Here's how the part is built. I have some questions about the finished solid (model axes, mm). Face numbers are marked on the shaded views. A direction names the side the tool comes from. Round coordinates to 2 decimals unless told otherwise and drop trailing zeros. Write each loop counter-clockwise with the first axis right and the second up, starting at its lowest first coordinate (ties: lowest second). Pieces come first, ordered by that corner, then holes. Notation, with made-up numbers: (57.5, -28) -> (93.5, -28) arc R13 ccw to (93.5, -3) -> close; hole circle Ø1 at (-1.5, 34.25). An arc over 180 degrees is marked (long way). Answer in a Markdown table with one row per item.
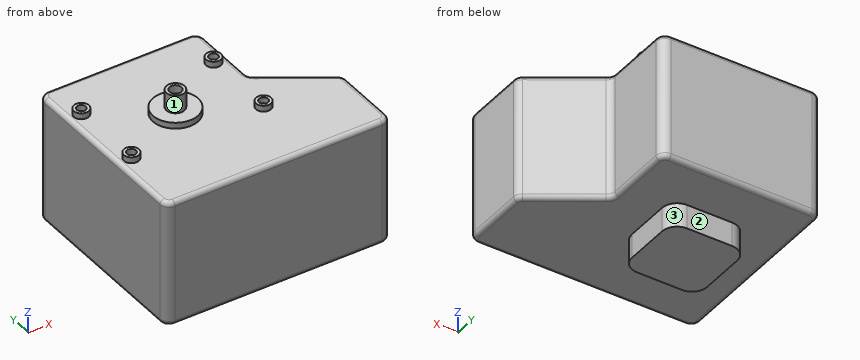
from build123d import *

# Parameters (mm, degrees)
BOSS_EXTRUDE1_DEPTH = 21
SKETCH3_R           = 2.5
SKETCH3_R_2         = 1.5
BOSS_EXTRUDE2_DEPTH = 2
SKETCH5_R           = 7.5
BOSS_EXTRUDE4_DEPTH = 2
FILLET1_R           = 3
FILLET2_R           = 1.5
SKETCH7_R           = 3
BOSS_EXTRUDE6_DEPTH = 6
SKETCH8_R           = 2
CUT_EXTRUDE2_DEPTH  = 77.552677941
BOSS_EXTRUDE7_DEPTH = 8


with BuildPart() as part:
    # Sketch2 → Boss-Extrude1 (new, symmetric)
    with BuildSketch(Plane.XY):
        Polygon((26.5, 6.75), (48.5, -7.75), (48.5, -31.75), (26.5, -31.75), (-26.5, -31.75), (-26.5, 31.75), (26.5, 31.75), align=None)
    extrude(amount=BOSS_EXTRUDE1_DEPTH, both=True)

    # Sketch3 → Boss-Extrude2 (add)
    # profile 1 of 4: a face of its own
    with BuildSketch(Plane.XY.offset(21)):
        with Locations(Location((-22, 17.25, 0), (0, 0, 180))):
            Circle(SKETCH3_R)
        with Locations((-22, 17.25)):
            Circle(SKETCH3_R_2, mode=Mode.SUBTRACT)
    # profile 2 of 4: a face of its own
    with BuildSketch(Plane.XY.offset(21)):
        with Locations(Location((22, 17.25, 0), (0, 0, 180))):
            Circle(SKETCH3_R)
        with Locations((22, 17.25)):
            Circle(SKETCH3_R_2, mode=Mode.SUBTRACT)
    # profile 3 of 4: a face of its own
    with BuildSketch(Plane.XY.offset(21)):
        with Locations(Location((-22, -7.75, 0), (0, 0, 180))):
            Circle(SKETCH3_R)
        with Locations((-22, -7.75)):
            Circle(SKETCH3_R_2, mode=Mode.SUBTRACT)
    # profile 4 of 4: a face of its own
    with BuildSketch(Plane.XY.offset(21)):
        with Locations(Location((22, -7.75, 0), (0, 0, 180))):
            Circle(SKETCH3_R)
        with Locations((22, -7.75)):
            Circle(SKETCH3_R_2, mode=Mode.SUBTRACT)
    extrude(amount=BOSS_EXTRUDE2_DEPTH)

    # Sketch5 → Boss-Extrude4 (add)
    with BuildSketch(Plane.XY.offset(21)):
        with Locations(Location((0, 3.25, 0), (0, 0, 180))):
            Circle(SKETCH5_R)
    extrude(amount=BOSS_EXTRUDE4_DEPTH)

    # Fillet1
    fillet1_edges = [part.edges().sort_by_distance(p)[0] for p in [
        (26.5, 6.75, 0),
        (48.5, -7.75, 0),
        (48.5, -31.75, 0),
        (-26.5, -31.75, 0),
        (-26.5, 31.75, 0),
        (26.5, 31.75, 0),
    ]]
    fillet(fillet1_edges, radius=FILLET1_R)

    # Fillet2
    fillet2_edges = [part.edges().sort_by_distance(p)[0] for p in [
        (11, -31.75, -21),
        (11, -31.75, 21),
        (26.5, 18.557860744, -21),
        (37.5, -0.5, -21),
        (48.5, -19.057860744, -21),
        (-26.5, 0, -21),
        (0, 31.75, -21),
        (25.621320344, 30.871320344, -21),
        (48.141289482, -7.943192097, -21),
        (47.621320344, -30.871320344, -21),
        (-25.621320344, 30.871320344, -21),
        (-25.621320344, -30.871320344, -21),
        (-26.5, 0, 21),
        (26.5, 18.557860744, 21),
        (0, 31.75, 21),
        (48.5, -19.057860744, 21),
        (37.5, -0.5, 21),
        (25.621320344, 30.871320344, 21),
        (48.141289482, -7.943192097, 21),
        (47.621320344, -30.871320344, 21),
        (-25.621320344, 30.871320344, 21),
        (-25.621320344, -30.871320344, 21),
        (26.858710518, 6.943192097, -21),
        (26.858710518, 6.943192097, 21),
    ]]
    fillet(fillet2_edges, radius=FILLET2_R)

    # Sketch7 → Boss-Extrude6 (add)
    with BuildSketch(Plane.XY.offset(23)):
        with Locations((0, 3.25)):
            Circle(SKETCH7_R)
    extrude(amount=BOSS_EXTRUDE6_DEPTH)

    # Sketch8 → Cut-Extrude2 (cut, through all)
    with BuildSketch(Plane.XY.offset(29)):
        with Locations((0, 3.25)):
            Circle(SKETCH8_R)
    extrude(amount=-CUT_EXTRUDE2_DEPTH, mode=Mode.SUBTRACT)

    # Sketch9 → Boss-Extrude7 (add)
    with BuildSketch(Plane(origin=(0, 0, -21), x_dir=(-1, 0, 0), z_dir=(0, 0, -1))):
        with BuildLine():
            Line((-7.5, -9.25), (7.5, -9.25))
            ThreePointArc((7.5, -9.25), (11.035533906, -7.785533906), (12.5, -4.25))
            Line((12.5, -4.25), (12.5, 10.75))
            ThreePointArc((12.5, 10.75), (11.035533906, 14.285533906), (7.5, 15.75))
            Line((7.5, 15.75), (-7.5, 15.75))
            ThreePointArc((-7.5, 15.75), (-11.035533906, 14.285533906), (-12.5, 10.75))
            Line((-12.5, 10.75), (-12.5, -4.25))
            ThreePointArc((-12.5, -4.25), (-11.035533906, -7.785533906), (-7.5, -9.25))
        make_face()
    extrude(amount=BOSS_EXTRUDE7_DEPTH)


solid = part.part
1) I want a section at D-D, the plane y = -17.5. List the corners of the cut face in (x, z) for me.
Response:
| item | result |
|---|---|
| outline | (-26.5, -19.5) arc R1.5 ccw to (-25, -21) -> (47, -21) arc R1.5 ccw to (48.5, -19.5) -> (48.5, 19.5) arc R1.5 ccw to (47, 21) -> (-25, 21) arc R1.5 ccw to (-26.5, 19.5) -> close |
2) For pin 1 (0.9 mm diameter, centred on x = 22, y = 17, fed in from +Z); pin 2 (2.5 mm diameter, centred on x = 21, y = -8.5, fed in from +Z); pin 3 (9 mm diameter, centred on x = 0.5, z = -26.5, fed in from -Y), each with a flat end and sliding along its axis, tell me the tip position at first contact or that it passes through.
Response:
| item | result |
|---|---|
| pin 1 | stops at z = 21 |
| pin 2 | stops at z = 23 |
| pin 3 | stops at y = -9.25 |
3) I want a section at C-C, the plane x = 0. List the corners of the cut face in (y, z) for me, and give its area (3 significant figures).
Response:
| item | result |
|---|---|
| outline | (-31.75, -19.5) arc R1.5 ccw to (-30.25, -21) -> (-9.25, -21) -> (-9.25, -29) -> (15.75, -29) -> (15.75, -21) -> (30.25, -21) arc R1.5 ccw to (31.75, -19.5) -> (31.75, 19.5) arc R1.5 ccw to (30.25, 21) -> (10.75, 21) -> (10.75, 23) -> (6.25, 23) -> (6.25, 29) -> (5.25, 29) -> (5.25, -21) -> (1.25, -21) -> (1.25, 29) -> (0.25, 29) -> (0.25, 23) -> (-4.25, 23) -> (-4.25, 21) -> (-30.25, 21) arc R1.5 ccw to (-31.75, 19.5) -> close |
| area | 2,730 mm^2 |
4) I want a section at B-B, the plane y = 17.25. List the corners of the cut face in (x, z) for me, and give its area (3 significant figures).
Response:
| item | result |
|---|---|
| outline | (-26.5, -19.5) arc R1.5 ccw to (-25, -21) -> (25, -21) arc R1.5 ccw to (26.5, -19.5) -> (26.5, 19.5) arc R1.5 ccw to (25, 21) -> (24.5, 21) -> (24.5, 23) -> (23.5, 23) -> (23.5, 21) -> (20.5, 21) -> (20.5, 23) -> (19.5, 23) -> (19.5, 21) -> (-19.5, 21) -> (-19.5, 23) -> (-20.5, 23) -> (-20.5, 21) -> (-23.5, 21) -> (-23.5, 23) -> (-24.5, 23) -> (-24.5, 21) -> (-25, 21) arc R1.5 ccw to (-26.5, 19.5) -> close |
| area | 2,230 mm^2 |
5) I want a section at A-A, the plane z = 1. List the corners of the cut face in (x, y) for me, and give its area (3 significant figures).
Response:
| item | result |
|---|---|
| outline | (-26.5, -28.75) arc R3 ccw to (-23.5, -31.75) -> (45.5, -31.75) arc R3 ccw to (48.5, -28.75) -> (48.5, -9.37) arc R3 ccw to (47.15, -6.86) -> (27.85, 5.86) arc R3 cw to (26.5, 8.37) -> (26.5, 28.75) arc R3 ccw to (23.5, 31.75) -> (-23.5, 31.75) arc R3 ccw to (-26.5, 28.75) -> close; hole circle Ø4 at (0, 3.25) |
| area | 4,030 mm^2 |
6) Which directions (+Z, -Z, +X, -X, +Y, -Y) give clear straight access to the entire face, cutting with the end or side of a thin tool? Please do the marked faces 1, 2 and 3.
Response:
| item | result |
|---|---|
| face 1 | +Z |
| face 2 | -Z, +X, -X, +Y |
| face 3 | -Z, +X, +Y |
7) I need wall thicknesses on line 1 (Z direction, x = -16.5, y = -28.5); line 2 (Z direction, x = -21.5, y = -5.5); line 3 (Y direction, x = 0, z = -10). Which ranges of each line are inside material? Lowest first, please. Write a range as [from, to].
Response:
| item | result |
|---|---|
| line 1 | z = [-21, 21] |
| line 2 | z = [-21, 23] |
| line 3 | y = [-31.75, 1.25], [5.25, 31.75] |
